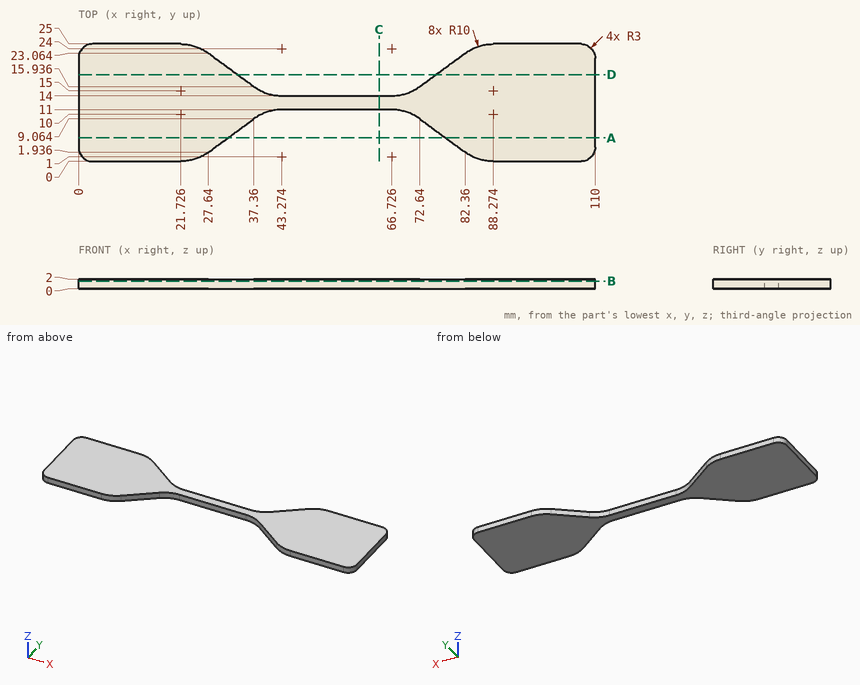
Study the drawing (mm; zero at the part's minimum x, y, z) and answer. Round coordinates to 2 decimals unless told otherwise and drop trailing zeros. Loops run counter-clockwise (first coordinate to the right, second up) from the corner with the lowest first, then second, coordinate; pieces in that order, holes last. Notation, with made-up numbers: (-17.5, 76) -> (34.5, 76) arc R24 cw to (34.5, 93) -> close; hole circle Ø7 at (22, -18). An arc over 180 degrees is marked (long way). Use one line per item in the form item = value.
1. The part is cut by section C-C on x = 64. Determine the outline of the cut face in (y, z).
Answer key:
outline = (11, 0) -> (14, 0) -> (14, 2) -> (11, 2) -> close
2. Flat-ended cylindrical pins translate along their axes: pin 1 Ø1 at (x, z) = (36.5, 1.5) entering from -Y; pin 2 Ø0.6 at (x, z) = (51, 1) entering from +Y. Find the tip coordinate at first contact, or state that the pin passes through.
Answer key:
pin_1 = 8.07
pin_2 = 14
3. The part is cut by section A-A on y = 5. Determine the outline of the cut face in (x, z), and give its area (3 significant figures).
Answer key:
outline = (0, 0) -> (31.82, 0) -> (31.82, 2) -> (0, 2) -> close; (78.18, 0) -> (110, 0) -> (110, 2) -> (78.18, 2) -> close
area = 127 mm²
4. The part is cut by section D-D on y = 18.5. Determine the outline of the cut face in (x, z).
Answer key:
outline = (0, 0) -> (33.86, 0) -> (33.86, 2) -> (0, 2) -> close; (76.14, 0) -> (110, 0) -> (110, 2) -> (76.14, 2) -> close
5. Find the intervals of material crossed by probe 1 along X at (y, z) = (5.75, 1.9); probe 2 along Y at (x, z) = (50, 0.7); probe 3 along X at (y, z) = (4.75, 0.8), in increasing order. Write a range as [from, to].
Answer key:
probe_1 = [0, 32.84], [77.16, 110]
probe_2 = [11, 14]
probe_3 = [0, 31.48], [78.52, 110]
6. The part is cut by section B-B on z = 1.65. Determine the outline of the cut face in (x, y).
Answer key:
outline = (0, 3) arc R3 ccw to (3, 0) -> (21.73, 0) arc R10 ccw to (27.64, 1.94) -> (37.36, 9.06) arc R10 cw to (43.27, 11) -> (66.73, 11) arc R10 cw to (72.64, 9.06) -> (82.36, 1.94) arc R10 ccw to (88.27, 0) -> (107, 0) arc R3 ccw to (110, 3) -> (110, 22) arc R3 ccw to (107, 25) -> (88.27, 25) arc R10 ccw to (82.36, 23.06) -> (72.64, 15.94) arc R10 cw to (66.73, 14) -> (43.27, 14) arc R10 cw to (37.36, 15.94) -> (27.64, 23.06) arc R10 ccw to (21.73, 25) -> (3, 25) arc R3 ccw to (0, 22) -> close
